from build123d import *

# Parameters (mm, degrees)
F0_R     = 0.5715
F1_DEPTH = 6.35


with BuildPart() as f1:
    # F0 (on Front) → F1 (new body)
    with BuildSketch(Plane.XZ):
        with BuildLine():
            ThreePointArc((23.241, 0), (21.086285, 6.564897), (14.176824, 6.559977))
            ThreePointArc((14.176824, 6.559977), (13.471175, 7.908419), (12.637654, 9.181793))
            ThreePointArc((12.637654, 9.181793), (13.480547, 14.50361), (18.802364, 13.660717))
            ThreePointArc((18.802364, 13.660717), (13.200413, 17.70532), (7.613434, 13.640061))
            ThreePointArc((7.613434, 13.640061), (6.249957, 14.316203), (4.827154, 14.856454))
            ThreePointArc((4.827154, 14.856454), (2.380984, 19.657334), (7.181864, 22.103504))
            ThreePointArc((7.181864, 22.103504), (0.272432, 22.082913), (-1.858029, 15.510105))
            ThreePointArc((-1.858029, 15.510105), (-3.358532, 15.255684), (-4.827154, 14.856454))
            ThreePointArc((-4.827154, 14.856454), (-9.628035, 17.302624), (-7.181864, 22.103504))
            ThreePointArc((-7.181864, 22.103504), (-12.759608, 18.025584), (-10.619788, 11.455817))
            ThreePointArc((-10.619788, 11.455817), (-11.684175, 10.368013), (-12.637654, 9.181793))
            ThreePointArc((-12.637654, 9.181793), (-17.959471, 8.3389), (-18.802364, 13.660717))
            ThreePointArc((-18.802364, 13.660717), (-20.917912, 7.083094), (-15.325149, 3.025796))
            ThreePointArc((-15.325149, 3.025796), (-15.546861, 1.520112), (-15.621, 0))
            ThreePointArc((-15.621, 0), (-19.431, -3.81), (-23.241, 0))
            ThreePointArc((-23.241, 0), (-21.086285, -6.564897), (-14.176824, -6.559977))
            ThreePointArc((-14.176824, -6.559977), (-13.471175, -7.908419), (-12.637654, -9.181793))
            ThreePointArc((-12.637654, -9.181793), (-13.480547, -14.50361), (-18.802364, -13.660717))
            ThreePointArc((-18.802364, -13.660717), (-13.200413, -17.70532), (-7.613434, -13.640061))
            ThreePointArc((-7.613434, -13.640061), (-6.249957, -14.316203), (-4.827154, -14.856454))
            ThreePointArc((-4.827154, -14.856454), (-2.380984, -19.657334), (-7.181864, -22.103504))
            ThreePointArc((-7.181864, -22.103504), (-0.272432, -22.082913), (1.858029, -15.510105))
            ThreePointArc((1.858029, -15.510105), (3.358532, -15.255684), (4.827154, -14.856454))
            ThreePointArc((4.827154, -14.856454), (9.628035, -17.302624), (7.181864, -22.103504))
            ThreePointArc((7.181864, -22.103504), (12.759608, -18.025584), (10.619788, -11.455817))
            ThreePointArc((10.619788, -11.455817), (11.684175, -10.368013), (12.637654, -9.181793))
            ThreePointArc((12.637654, -9.181793), (17.959471, -8.3389), (18.802364, -13.660717))
            ThreePointArc((18.802364, -13.660717), (20.917912, -7.083094), (15.325149, -3.025796))
            ThreePointArc((15.325149, -3.025796), (15.546861, -1.520112), (15.621, 0))
            ThreePointArc((15.621, 0), (19.431, 3.81), (23.241, 0))
        make_face()
        Circle(F0_R, mode=Mode.SUBTRACT)
    extrude(amount=F1_DEPTH)


solid = f1.part
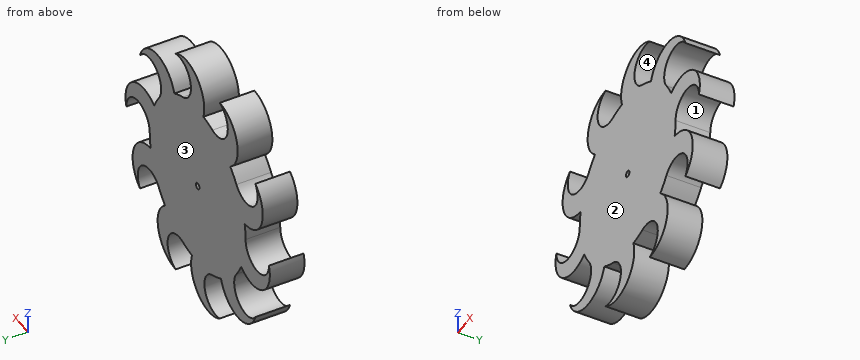
Could you check a few things on this model? Use its own coordinates, in mm. Face numbers are marked on the shaded views. A direction names the side the tool comes from. Give positions to 0.01 mm unless a question says otherwise; leave off trailing zeros. Order: outer loops, then holes, each group sorted by start corner. A loop starts at its lowest first (then second) coordinate and runs counter-clockwise, first axis right, second up. Notation, with made-up numbers: (72, -26.75) - (103, -26.75) arc R16 cw to (103, -13.75) - close; hole circle Ø11 at (83.5, 27). An arc over 180 degrees is marked (long way). Return JSON: item names as keys, results as strings. Group by question number.
Q1. Which directions (+Z, -Z, +X, -X, +Y, -Y) give clear straight access to the entire face, cutting with the end or side of a thin tool? Please do the marked faces 1 and 2.
Q2. Thinking about a two-plate mould opening in Z: for the marked faces 3 and 4, which applies, pulls with the +Z half, pulls with the -Z half, needs draft (parallel to the pull), parting line crosses it, or undercut?
Q3. Please list where these lines run through material, in increasing order: line 1 along Z through (x, y) = (-16.5, -4.25); line 2 along X through (y, z) = (-4.75, -8.5); line 3 along Z through (x, y) = (0, -2.75). Write a range as [from, to].
Q4. Suppose I cut it at B-B, the plane x = -4. Please give me the cut outline in (y, z).
Q5. Will this pin go through, and if not, where does the flat tip stop? pin 1 Ø1 at (y, z) = (-3.5, -9) entering from -X.
Q6. Suppose I cut it at C-C, the plane z = -13. Please give me the cut outline in (x, y).
Resolved:
{
 "1": {"face 1": "+Y, -Y", "face 2": "+Z, -Z, +X, -X, -Y"},
 "2": {"face 3": "needs draft", "face 4": "undercut"},
 "3": {"line 1": "z = [-16.7, -15.15], [-7.57, -2.43], [3.14, 7.69]", "line 2": "x = [-13.11, 13.27], [18.17, 21.19]", "line 3": "z = [-21.87, -0.57], [0.57, 21.87]"},
 "4": {"outline": "(-6.35, -23.21) - (0, -23.21) - (0, -21.72) - (-6.35, -21.72) - close; (-6.35, -15.24) - (0, -15.24) - (0, 15.1) - (-6.35, 15.1) - close"},
 "5": {"pin 1": "stops at x = -13.11"},
 "6": {"outline": "(-12.25, -6.35) - (12.09, -6.35) - (12.09, 0) - (-12.25, 0) - close; (19.19, -6.35) - (19.56, -6.35) - (19.56, 0) - (19.19, 0) - close"}
}
